Can you work these out from the model? Positions are in its coordinate system, mm. Face numbers are marked on the shaded views. A direction names the side the tool comes from. Give positions to 0.01 mm unless a question says otherwise; leave off trailing zeros. Loops run counter-clockwise (first coordinate to the right, second up) from the corner with the lowest first, then second, coordinate; pieces in that order, holes last. Notation, with made-up numbers: (38, 0) - (47, 0) arc R10 ccw to (47, 4) - close; hole circle Ø2 at (27.25, 13). An arc over 180 degrees is marked (long way). Answer as a JSON object with one key per item and string values.
```python
from build123d import *

# Parameters (mm, degrees)
F0_W     = 480
F0_H     = 300
F1_DEPTH = 620
F2_T     = -3
F4_DEPTH = 362


with BuildPart() as f1:
    # F0 (on Top) → F1 (new body)
    with BuildSketch(Plane.XY):
        Rectangle(F0_W, F0_H)
    extrude(amount=F1_DEPTH)

    # F2
    f2_openings = [f1.faces().sort_by_distance(p)[0] for p in [
        (0, 0, 620),
    ]]
    offset(amount=F2_T, openings=f2_openings)

    # F3 (on Right) → F4 (cut, symmetric)
    with BuildSketch(Plane.YZ):
        with BuildLine():
            Line((-208.315447, 59.702795), (-150, 59.702795))
            Line((-150, 59.702795), (-147, 59.702795))
            Line((-147, 59.702795), (-74.486937, 498.891666))
            ThreePointArc((-74.486937, 498.891666), (-66.749185, 516.734135), (-51.511216, 528.818454))
            Line((-51.511216, 528.818454), (150, 620))
            Line((150, 620), (136.103183, 668.386102))
            Line((136.103183, 668.386102), (-228.213415, 668.386102))
            Line((-228.213415, 668.386102), (-208.315447, 59.702795))
        make_face()
    extrude(amount=F4_DEPTH, both=True, mode=Mode.SUBTRACT)


solid = f1.part
```
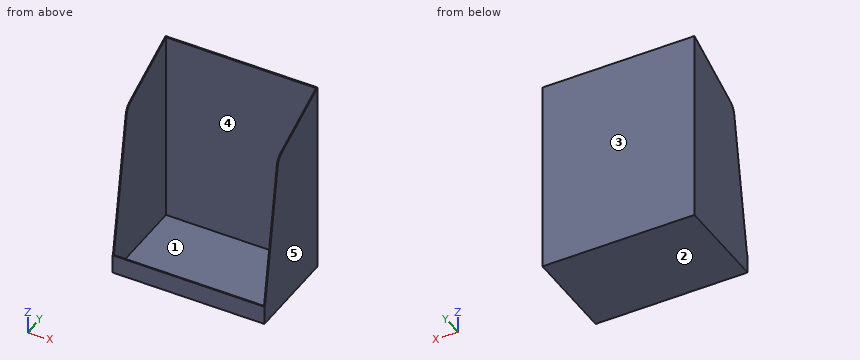
1) If we mould it in two halves opening along X, with no side actions, what happens to the marked faces 3, 4 and 5? For each: released by +X, released by -X, zero draft, split by the parting line, or undercut.
Check sheet entries:
{"face 3": "zero draft", "face 4": "undercut", "face 5": "released by +X"}
2) Which directions (+Z, -Z, +X, -X, +Y, -Y) give clear straight access to the entire face, cutting with the end or side of a thin tool? Please do the marked faces 1 and 2.
Check sheet entries:
{"face 1": "+Z", "face 2": "-Z, +X, -X, +Y, -Y"}
3) I need wall thicknesses on L1, parallel to X at y = 10, z = 210.5; L2, parallel to Y at x = -79, z = 56; L3, parallel to Y at x = -170, z = 309.5. Which ranges of each line are inside material? Lowest first, please.
Check sheet entries:
{"L1": "-240 to -237, 237 to 240", "L2": "-150 to -147, 147 to 150", "L3": "147 to 150"}
4) Imagine slicing it at B-B on z = 361.5. Write out the boundary of the cut face in (x, y), and give its area (3 significant figures).
Check sheet entries:
{"outline": "(-240, -97.17) - (-237, -97.17) - (-237, 147) - (237, 147) - (237, -97.17) - (240, -97.17) - (240, 150) - (-240, 150) - close", "area": "2,910 mm2"}
5) I'm going to push flat-ended pins straight in: P1, Ø1.5, axis at x = -21, y = -149, coming from the +Z side; P2, Ø6, axis at x = -7.5, y = -58, coming from the +Z side. Where does each tip first touch, or does it pass through?
Check sheet entries:
{"P1": "z = 59.7", "P2": "z = 3"}
6) Imagine slicing it at A-A on x = 4. Write out the boundary of the cut face in (y, z), and give its area (3 significant figures).
Check sheet entries:
{"outline": "(-150, 0) - (150, 0) - (150, 620) - (147, 618.64) - (147, 3) - (-147, 3) - (-147, 59.7) - (-150, 59.7) - close", "area": "2,920 mm2"}
